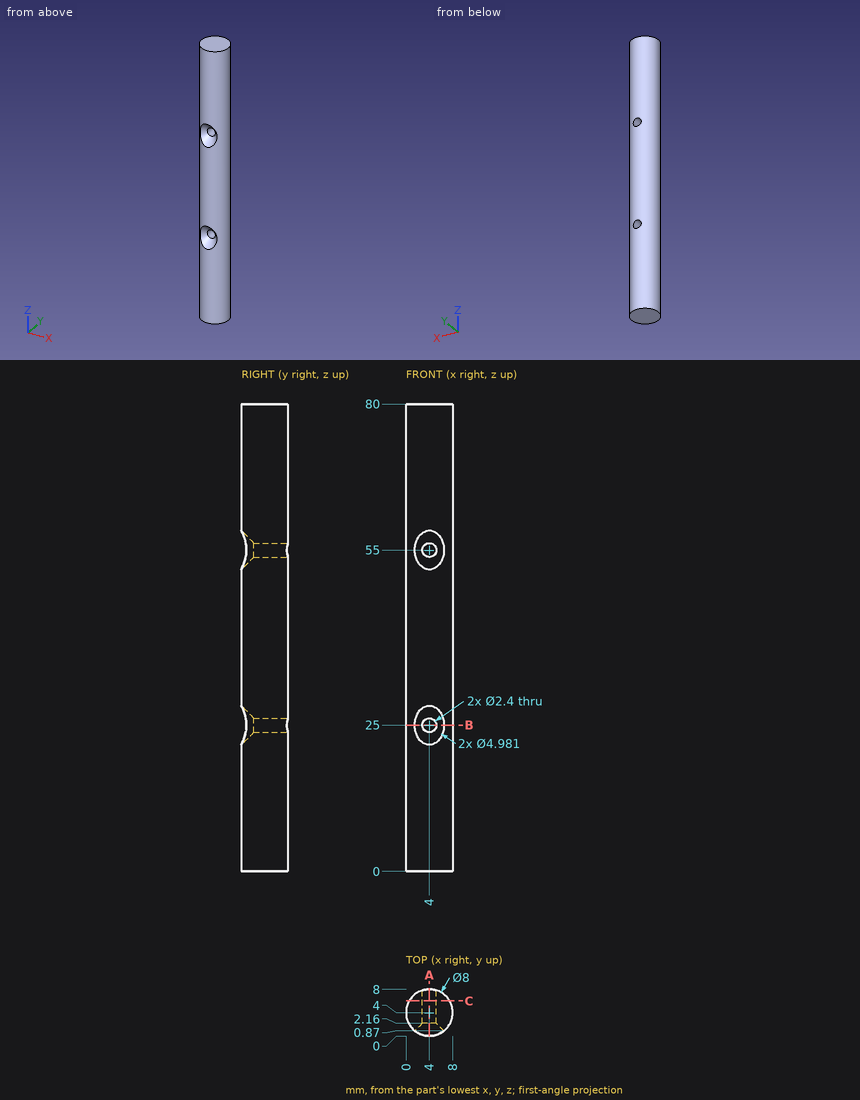
Part print with two shaded views. Sizes in mm from the minimum x, y, z corner. Round coordinates to 2 decimals unless told otherwise and drop trailing zeros. Order: outer loops, then holes, each group sorted by start corner. A loop starts at its lowest first (then second) coordinate and runs counter-clockwise, first axis right, second up. Notation, with made-up numbers: (-15, 33.5) - (26, 33.5) arc R28 cw to (26, 61.5) - close; hole circle Ø3 at (32, -1.75). An arc over 180 degrees is marked (long way). Answer as CSV lines item,"result". Start each with the question number.
1. Saw through at A-A, the plane x = 4. Write the cut outline in (y, z), and give its area (3 significant figures).
2. Saw through at C-C, the plane y = 6. Write the cut outline in (x, z) (1 decimal).
3. Pin check, flat tips, straight feed: pin 1 (1.4 mm diameter, centred on x = 4, z = 55, fed in from +Y); pin 2 (3 mm diameter, centred on x = 4, z = 25, fed in from -Y); pin 3 (4 mm diameter, centred on y = 3, z = 28.5, fed in from -X); pin 4 (3 mm diameter, centred on y = 6.5, z = 18, fed in from +X). Stop position of each tip, or through.
4. Saw through at B-B, the plane z = 25. Write the cut outline in (x, y) (1 decimal).
5. Drill centre lines: L1, parallel to Z at x = 4, y = 5.8; L2, parallel to Z at x = 3, y = 3.75 (1 decimal); L3, parallel to X at y = 3.75, z = 33. Where is each one in solid material? Low to high. Write a range as [from, to].
Model answer:
1,outline,"(0, 0) - (8, 0) - (8, 23.8) - (2.16, 23.8) - (0, 21.64) - close; (0, 28.36) - (2.16, 26.2) - (8, 26.2) - (8, 53.8) - (2.16, 53.8) - (0, 51.64) - close; (0, 58.36) - (2.16, 56.2) - (8, 56.2) - (8, 80) - (0, 80) - close"
1,area,"592 mm²"
2,outline,"(0.5, 0) - (7.5, 0) - (7.5, 80) - (0.5, 80) - close; hole circle Ø2.4 at (4, 25); hole circle Ø2.4 at (4, 55)"
3,pin 1,"passes through"
3,pin 2,"stops at y = 1.86"
3,pin 3,"stops at x = 0"
3,pin 4,"stops at x = 7.87"
4,outline,"(1.5, 0.9) - (2.8, 2.2) - (2.8, 7.8) arc R4 ccw to start; (5.2, 2.2) - (6.5, 0.9) arc R4 ccw to (5.2, 7.8) - close"
5,L1,"z = [0, 23.8], [26.2, 53.8], [56.2, 80]"
5,L2,"z = [0, 24.3], [25.7, 54.3], [55.7, 80]"
5,L3,"x = [0.01, 7.99]"
